Geometry: final body of the model. Coordinates: model frame, mm. A direction names the side the tool comes from. Round coordinates to 2 decimals unless told otherwise and drop trailing zeros. Loops run counter-clockwise (first coordinate to the right, second up) from the corner with the lowest first, then second, coordinate; pieces in that order, holes last. Notation, with made-up numbers: (47, 45) - (69, 45) arc R20 cw to (69, 64) - close; hole circle Ø9 at (67, -2.75). An arc over 180 degrees is marked (long way). Write item = value, one per line. Start each with the question number.
Item 1: Line query: line 1 (X direction, y = -4.5, z = -14); line 2 (Y direction, x = -37, z = -22.25); line 3 (X direction, y = -26.5, z = -10). Output: solid intervals per line, ascending. Write a range as from..to.
Item 2: Section B-B (y = 12). Return loops of the section in (x, z).
Item 3: Draft query along X for faces 1 (the conical face through (-50.252, 27.249, -3.395)), 2 (the flat face through (-55.596, -1, -13)), 3 (the cylindrical face through (-4.32, 34.29, -0.57)), 4 (the cylindrical face through (-57.025, -34.507, -13.339)). Return one class per face: pulls with the +X half, pulls with the -X half, needs draft (parallel to the pull), parting line crosses it, or undercut.
Item 4: Section C-C (z = -10.25). Count the separate pieces of the cut face and the enclosed holes in it, plus the area to 3 significant figures.
Item 5: First-contact query: pin 1 (1 mm diameter, centred on y = 34, z = -24, fed in from -X); pin 2 (20.5 mm diameter, centred on x = -27, y = 11.5, fed in from -Z); pin 3 (3 mm diameter, centred on x = 42.5, y = -27.5, fed in from -Z). Flat tips, straight axial feed; report the tip coordinate or a pass-through.
Item 6: Section A-A (x = 6.5). Return loops of the section in (y, z).
Item 7: Section D-D (z = -16.5). Return loops of the section in (x, y), plus the area to 3 significant figures.
Item 8: Access query for faces 5 (the cylindrical face through (25.5, -34.1, -18.5)), 6 (the flat face through (-50, 26, -14)), 7 (the cylindrical face through (49.8, 0.35, -0.57)), 8 (the flat face through (-43.596, 1, -1)). Directions: +Z, -Z, +X, -X, +Y, -Y. A direction counts if a zero-diameter tool reaches every point of the face in a straight line with its end or side. Return the directions, or none.
from build123d import *

# Parameters (mm, degrees)
F0_W      = 104
F0_H      = 66
F0_R      = 3
F1_DEPTH  = 2
F2_DEPTH  = 22.49
F3_DEPTH  = 23
F4_DEPTH  = 14
F6_DEPTH  = 2.5
F7_W      = 21
F7_H      = 2.4
F8_DEPTH  = 2.5
F10_D     = 2.4384
F10_DEPTH = 10
F10_TIP   = 0.7325692667
F11_R     = 2
F12_R     = 1


with BuildPart() as f1:
    # F0 (on Top) → F1 (new body)
    with BuildSketch(Plane.XY):
        with BuildLine():
            Line((48.4044117422, 34.8920698583), (-55.5955882578, 34.8920698583))
            ThreePointArc((-55.5955882578, 34.8920698583), (-57.0098018202, 34.3062834207), (-57.5955882578, 32.8920698583))
            Line((-57.5955882578, 32.8920698583), (-57.5955882578, -33.1079301417))
            ThreePointArc((-57.5955882578, -33.1079301417), (-57.0098018202, -34.5221437041), (-55.5955882578, -35.1079301417))
            Line((-55.5955882578, -35.1079301417), (48.4044117422, -35.1079301417))
            ThreePointArc((48.4044117422, -35.1079301417), (49.8186253046, -34.5221437041), (50.4044117422, -33.1079301417))
            Line((50.4044117422, -33.1079301417), (50.4044117422, 32.8920698583))
            ThreePointArc((50.4044117422, 32.8920698583), (49.8186253046, 34.3062834207), (48.4044117422, 34.8920698583))
        make_face()
        with BuildLine():
            ThreePointArc((-56.6455882578, 32.8920698583), (-56.338050378, 33.6345319786), (-55.5955882578, 33.9420698583))
            Line((-55.5955882578, 33.9420698583), (48.4044117422, 33.9420698583))
            ThreePointArc((48.4044117422, 33.9420698583), (49.1468738625, 33.6345319786), (49.4544117422, 32.8920698583))
            Line((49.4544117422, 32.8920698583), (49.4544117422, -33.1079301417))
            ThreePointArc((49.4544117422, -33.1079301417), (49.1468738625, -33.8503922619), (48.4044117422, -34.1579301417))
            Line((48.4044117422, -34.1579301417), (-55.5955882578, -34.1579301417))
            ThreePointArc((-55.5955882578, -34.1579301417), (-56.338050378, -33.8503922619), (-56.6455882578, -33.1079301417))
            Line((-56.6455882578, -33.1079301417), (-56.6455882578, 32.8920698583))
        make_face(mode=Mode.SUBTRACT)
        with BuildLine():
            Line((48.4044117422, 33.9420698583), (-55.5955882578, 33.9420698583))
            ThreePointArc((-55.5955882578, 33.9420698583), (-56.338050378, 33.6345319786), (-56.6455882578, 32.8920698583))
            Line((-56.6455882578, 32.8920698583), (-56.6455882578, -33.1079301417))
            ThreePointArc((-56.6455882578, -33.1079301417), (-56.338050378, -33.8503922619), (-55.5955882578, -34.1579301417))
            Line((-55.5955882578, -34.1579301417), (48.4044117422, -34.1579301417))
            ThreePointArc((48.4044117422, -34.1579301417), (49.1468738625, -33.8503922619), (49.4544117422, -33.1079301417))
            Line((49.4544117422, -33.1079301417), (49.4544117422, 32.8920698583))
            ThreePointArc((49.4544117422, 32.8920698583), (49.1468738625, 33.6345319786), (48.4044117422, 33.9420698583))
        make_face()
        with Locations((-3.5955882578, -0.1079301417)):
            Rectangle(F0_W, F0_H, mode=Mode.SUBTRACT)
        with Locations((-3.5955882578, -0.1079301417)):
            Rectangle(F0_W, F0_H)
        with Locations((-50.0955882578, -27.6079301417)):
            Circle(F0_R, mode=Mode.SUBTRACT)
        with Locations((42.9044117422, -27.6079301417)):
            Circle(F0_R, mode=Mode.SUBTRACT)
        with Locations((-50.0955882578, 27.3920698583)):
            Circle(F0_R, mode=Mode.SUBTRACT)
        with BuildLine():
            ThreePointArc((-43.5955882578, 13.4650188752), (-44.424068371, 16.2812101433), (-41.5144494277, 15.8920698583))
            Line((-41.5144494277, 15.8920698583), (34.3232729121, 15.8920698583))
            ThreePointArc((34.3232729121, 15.8920698583), (36.2887989476, 16.8493327192), (37.6544117422, 15.1420698583))
            ThreePointArc((37.6544117422, 15.1420698583), (37.3075332623, 14.0962448251), (36.4044117422, 13.4650188752))
            Line((36.4044117422, 13.4650188752), (36.4044117422, -11.6808791586))
            ThreePointArc((36.4044117422, -11.6808791586), (37.3075332623, -12.3121051085), (37.6544117422, -13.3579301417))
            ThreePointArc((37.6544117422, -13.3579301417), (36.2887989476, -15.0651930026), (34.3232729121, -14.1079301417))
            Line((34.3232729121, -14.1079301417), (-41.5144494277, -14.1079301417))
            ThreePointArc((-41.5144494277, -14.1079301417), (-44.424068371, -14.4970704267), (-43.5955882578, -11.6808791586))
            Line((-43.5955882578, -11.6808791586), (-43.5955882578, 13.4650188752))
        make_face(mode=Mode.SUBTRACT)
        with Locations((42.9044117422, 27.3920698583)):
            Circle(F0_R, mode=Mode.SUBTRACT)
        with Locations((-50.0955882578, 27.3920698583)):
            Circle(F0_R)
        with Locations((42.9044117422, 27.3920698583)):
            Circle(F0_R)
        with Locations((42.9044117422, -27.6079301417)):
            Circle(F0_R)
        with Locations((-50.0955882578, -27.6079301417)):
            Circle(F0_R)
    extrude(amount=-F1_DEPTH)

    # F0 (on Top) → F2 (join)
    with BuildSketch(Plane.XY):
        with BuildLine():
            Line((48.4044117422, 33.9420698583), (-55.5955882578, 33.9420698583))
            ThreePointArc((-55.5955882578, 33.9420698583), (-56.338050378, 33.6345319786), (-56.6455882578, 32.8920698583))
            Line((-56.6455882578, 32.8920698583), (-56.6455882578, -33.1079301417))
            ThreePointArc((-56.6455882578, -33.1079301417), (-56.338050378, -33.8503922619), (-55.5955882578, -34.1579301417))
            Line((-55.5955882578, -34.1579301417), (48.4044117422, -34.1579301417))
            ThreePointArc((48.4044117422, -34.1579301417), (49.1468738625, -33.8503922619), (49.4544117422, -33.1079301417))
            Line((49.4544117422, -33.1079301417), (49.4544117422, 32.8920698583))
            ThreePointArc((49.4544117422, 32.8920698583), (49.1468738625, 33.6345319786), (48.4044117422, 33.9420698583))
        make_face()
        with Locations((-3.5955882578, -0.1079301417)):
            Rectangle(F0_W, F0_H, mode=Mode.SUBTRACT)
    extrude(amount=-F2_DEPTH)

    # F3 (add): a face of the model
    f3_faces = [f1.faces().sort_by_distance(p)[0] for p in [
        (-3.5955882578, 34.763368654, -2),
    ]]
    extrude(f3_faces, amount=F3_DEPTH)

    # F0 (on Top) → F4 (join)
    with BuildSketch(Plane.XY):
        with Locations((-50.0955882578, 27.3920698583)):
            Circle(F0_R)
        with Locations((42.9044117422, 27.3920698583)):
            Circle(F0_R)
        with Locations((-50.0955882578, -27.6079301417)):
            Circle(F0_R)
        with Locations((42.9044117422, -27.6079301417)):
            Circle(F0_R)
    extrude(amount=-F4_DEPTH)

    # F5 (on face) → F6 (cut)
    with BuildSketch(Plane.XZ.offset(35.1079301417)):
        with BuildLine():
            Line((18.9044117422, -25), (31.9044117422, -25))
            ThreePointArc((31.9044117422, -25), (25.4044117422, -18.5), (18.9044117422, -25))
        make_face()
    extrude(amount=-F6_DEPTH, mode=Mode.SUBTRACT)

    # F7 (on face) → F8 (cut)
    with BuildSketch(Plane(origin=(0, 34.8920698583, 0), x_dir=(-1, 0, 0), z_dir=(0, 1, 0))):
        with Locations((-18.3044117422, -23.8)):
            Rectangle(F7_W, F7_H)
    extrude(amount=-F8_DEPTH, mode=Mode.SUBTRACT)

    # F10
    with Locations(Plane(origin=(0, 0, -14), x_dir=(1, 0, 0), z_dir=(0, 0, -1))):
        with Locations((-50.0955882578, -27.3920698583), (42.9044117422, -27.3920698583), (42.9044117422, 27.6079301417), (-50.0955882578, 27.6079301417)):
            Hole(F10_D / 2, depth=F10_DEPTH)
            with Locations((0, 0, -(F10_DEPTH + F10_TIP / 2))):  # 118° drill point
                Cone(0, F10_D / 2, F10_TIP, mode=Mode.SUBTRACT)

    # F11
    f11_edges = [f1.edges().sort_by_distance(p)[0] for p in [
        (-57.595588, -0.10793, 0),
        (-3.595588, 34.89207, 0),
        (50.404412, -0.10793, 0),
        (-3.595588, -35.10793, 0),
        (-57.009802, 34.306283, 0),
        (-57.009802, -34.522144, 0),
        (49.818625, -34.522144, 0),
        (49.818625, 34.306283, 0),
    ]]
    fillet(f11_edges, radius=F11_R)

    # F12
    f12_edges = [f1.edges().sort_by_distance(p)[0] for p in [
        (48.404412, -33.10793, -12.245),
        (48.404412, -0.10793, -2),
        (-3.595588, -33.10793, -2),
        (-55.595588, -33.10793, -12.245),
        (-55.595588, -0.10793, -2),
        (-55.595588, 32.89207, -12.245),
        (-3.595588, 32.89207, -2),
        (48.404412, 32.89207, -12.245),
    ]]
    fillet(f12_edges, radius=F12_R)


solid = f1.part
Taken from the geometry:
q1.line_1 = -57.6..-55.6, 48.4..50.4
q1.line_2 = -35.11..-33.11, 32.89..34.89
q1.line_3 = -57.6..-55.6, -52.88..-50.6, -49.59..-47.31, 40.12..42.4, 43.41..45.69, 48.4..50.4
q2.outline = (-57.6, -25) - (-56.65, -25) - (-56.65, -22.49) - (-55.6, -22.49) - (-55.6, -3) arc R1 cw to (-54.6, -2) - (-43.6, -2) - (-43.6, 0) - (-55.6, 0) arc R2 ccw to (-57.6, -2) - close; (36.4, -2) - (47.4, -2) arc R1 cw to (48.4, -3) - (48.4, -22.49) - (49.45, -22.49) - (49.45, -25) - (50.4, -25) - (50.4, -2) arc R2 ccw to (48.4, 0) - (36.4, 0) - close
q3.face_1 = undercut
q3.face_2 = undercut
q3.face_3 = needs draft
q3.face_4 = pulls with the -X half
q4.separate_pieces = 5
q4.enclosed_holes = 5
q4.area = 788 mm^2
q5.pin_1 = -57.5
q5.pin_2 = -2
q5.pin_3 = -14
q6.outline = (-35.11, -25) - (-34.16, -25) - (-34.16, -22.49) - (-33.11, -22.49) - (-33.11, -3) arc R1 cw to (-32.11, -2) - (-14.11, -2) - (-14.11, 0) - (-33.11, 0) arc R2 ccw to (-35.11, -2) - close; (15.89, -2) - (31.89, -2) arc R1 cw to (32.89, -3) - (32.89, -22.49) - (33.94, -22.49) - (33.94, -25) - (34.89, -25) - (34.89, -2) arc R2 ccw to (32.89, 0) - (15.89, 0) - close
q7.outline = (-57.6, -33.11) arc R2 ccw to (-55.6, -35.11) - (48.4, -35.11) arc R2 ccw to (50.4, -33.11) - (50.4, 32.89) arc R2 ccw to (48.4, 34.89) - (-55.6, 34.89) arc R2 ccw to (-57.6, 32.89) - close; hole (-55.6, -32.11) arc R1 ccw to (-54.6, -33.11) - (47.4, -33.11) arc R1 ccw to (48.4, -32.11) - (48.4, 31.89) arc R1 ccw to (47.4, 32.89) - (-54.6, 32.89) arc R1 ccw to (-55.6, 31.89) - close
q7.area = 693 mm^2
q8.face_5 = -Z, -Y
q8.face_6 = -Z
q8.face_7 = +Z, +X, +Y, -Y
q8.face_8 = +Z, -Z
